Input: part model. Units: mm. Frame: model coordinates. A direction names the side the tool comes from. Give positions to 0.01 mm unless a question says otherwise; leave off trailing zeros. Loops run counter-clockwise (first coordinate to the right, second up) from the corner with the lowest first, then second, coordinate; pieces in that order, holes last. Notation, with made-up numbers: M -15.5,-6 L 34.5,-6 A24 ccw 34.5,4 Z; hole C 81,-32.75 d5. An arc over 180 degrees is marked long. Answer as a JSON object with one key per item and string values. Group by question number.
1) Section query B-B on y = 16.5. Return loops of the section in (x, z).
2) Section query C-C on z = -11. Return loops of the section in (x, y), plus the area to 3 significant figures.
3) Access query for faces 4 (the flat face through (11, 35, 0)), 5 (the flat face through (1, 35, -11)). Directions: +Z, -Z, +X, -X, +Y, -Y. A direction counts if a zero-diameter tool reaches every point of the face in a straight line with its end or side. Return the directions, or none.
4) Ray query, L1, parallel to Y at x = 11, z = -0.8; L2, parallel to X at y = 29.5, z = -7.75; L3, parallel to Z at x = 15.5, y = 45.5. Return the intervals inside material, ascending.
5) Section query D-D on z = -6. Return loops of the section in (x, y), plus the area to 3 significant figures.
6) Section query A-A on x = 11. Return loops of the section in (y, z).
7) Draft query along Z for faces 1 (the cylindrical face through (0.507, 18.483, -10.74)), 2 (the flat face through (11, 35, -1)), 3 (the flat face through (5.9, 70, -0.4)). Return one class per face: +Z half, -Z half, draft (parallel to the pull), parting line (faces both ways), or undercut.
8) First-contact query: P1, Ø5, axis at x = 11, y = 6.5, coming from the +Z side; P2, Ø6.5, axis at x = 11, y = 63.5, coming from the -Z side; P3, Ø1.5, axis at y = 11.5, z = -7, coming from the +X side. Flat tips, straight axial feed; report the tip coordinate or a pass-through.
from build123d import *

# Parameters (mm, degrees)
EXTRUSION1_DEPTH = 70
EXTRUSION2_REACH = 3
ESQUISSE2_R      = 2
EXTRUSION3_REACH = 3
ESQUISSE3_R      = 2


with BuildPart() as part:
    # Esquisse1 → Extrusion1 (new body)
    with BuildSketch(Plane(origin=(0, 0, 0), x_dir=(1, 0, 0), z_dir=(0, 1, 0))):
        Polygon((0, 0), (0, 21), (1, 21), (1, 1), (21, 1), (21, 0), align=None)
    extrude(amount=EXTRUSION1_DEPTH)

    # Esquisse2 → Extrusion2 (cut, up to next)
    with BuildSketch(Plane(origin=(1, 0, 0), x_dir=(0, 0, -1), z_dir=(1, 0, 0)), mode=Mode.PRIVATE) as extrusion2_sk1:
        with Locations((11, 16.5)):
            Circle(ESQUISSE2_R)
    extrusion2_tool1 = extrude(extrusion2_sk1.sketch, amount=-EXTRUSION2_REACH, mode=Mode.PRIVATE) & part.part
    add(extrusion2_tool1.solids().sort_by_distance((1, 16.5, -11))[0], mode=Mode.SUBTRACT)
    # Esquisse2 → Extrusion2 (cut, up to next)
    with BuildSketch(Plane(origin=(1, 0, 0), x_dir=(0, 0, -1), z_dir=(1, 0, 0)), mode=Mode.PRIVATE) as extrusion2_sk2:
        with Locations((11, 6.5)):
            Circle(ESQUISSE2_R)
    extrusion2_tool2 = extrude(extrusion2_sk2.sketch, amount=-EXTRUSION2_REACH, mode=Mode.PRIVATE) & part.part
    add(extrusion2_tool2.solids().sort_by_distance((1, 6.5, -11))[0], mode=Mode.SUBTRACT)
    # Esquisse2 → Extrusion2 (cut, up to next)
    with BuildSketch(Plane(origin=(1, 0, 0), x_dir=(0, 0, -1), z_dir=(1, 0, 0)), mode=Mode.PRIVATE) as extrusion2_sk3:
        with Locations((11, 53.5)):
            Circle(ESQUISSE2_R)
    extrusion2_tool3 = extrude(extrusion2_sk3.sketch, amount=-EXTRUSION2_REACH, mode=Mode.PRIVATE) & part.part
    add(extrusion2_tool3.solids().sort_by_distance((1, 53.5, -11))[0], mode=Mode.SUBTRACT)
    # Esquisse2 → Extrusion2 (cut, up to next)
    with BuildSketch(Plane(origin=(1, 0, 0), x_dir=(0, 0, -1), z_dir=(1, 0, 0)), mode=Mode.PRIVATE) as extrusion2_sk4:
        with Locations((11, 63.5)):
            Circle(ESQUISSE2_R)
    extrusion2_tool4 = extrude(extrusion2_sk4.sketch, amount=-EXTRUSION2_REACH, mode=Mode.PRIVATE) & part.part
    add(extrusion2_tool4.solids().sort_by_distance((1, 63.5, -11))[0], mode=Mode.SUBTRACT)

    # Esquisse3 → Extrusion3 (cut, up to next)
    with BuildSketch(Plane(origin=(0, 0, -1), x_dir=(-1, 0, 0), z_dir=(0, 0, -1)), mode=Mode.PRIVATE) as extrusion3_sk1:
        with Locations((-11, 53.5)):
            Circle(ESQUISSE3_R)
    extrusion3_tool1 = extrude(extrusion3_sk1.sketch, amount=-EXTRUSION3_REACH, mode=Mode.PRIVATE) & part.part
    add(extrusion3_tool1.solids().sort_by_distance((11, 53.5, -1))[0], mode=Mode.SUBTRACT)
    # Esquisse3 → Extrusion3 (cut, up to next)
    with BuildSketch(Plane(origin=(0, 0, -1), x_dir=(-1, 0, 0), z_dir=(0, 0, -1)), mode=Mode.PRIVATE) as extrusion3_sk2:
        with Locations((-11, 63.5)):
            Circle(ESQUISSE3_R)
    extrusion3_tool2 = extrude(extrusion3_sk2.sketch, amount=-EXTRUSION3_REACH, mode=Mode.PRIVATE) & part.part
    add(extrusion3_tool2.solids().sort_by_distance((11, 63.5, -1))[0], mode=Mode.SUBTRACT)
    # Esquisse3 → Extrusion3 (cut, up to next)
    with BuildSketch(Plane(origin=(0, 0, -1), x_dir=(-1, 0, 0), z_dir=(0, 0, -1)), mode=Mode.PRIVATE) as extrusion3_sk3:
        with Locations((-11, 6.5)):
            Circle(ESQUISSE3_R)
    extrusion3_tool3 = extrude(extrusion3_sk3.sketch, amount=-EXTRUSION3_REACH, mode=Mode.PRIVATE) & part.part
    add(extrusion3_tool3.solids().sort_by_distance((11, 6.5, -1))[0], mode=Mode.SUBTRACT)
    # Esquisse3 → Extrusion3 (cut, up to next)
    with BuildSketch(Plane(origin=(0, 0, -1), x_dir=(-1, 0, 0), z_dir=(0, 0, -1)), mode=Mode.PRIVATE) as extrusion3_sk4:
        with Locations((-11, 16.5)):
            Circle(ESQUISSE3_R)
    extrusion3_tool4 = extrude(extrusion3_sk4.sketch, amount=-EXTRUSION3_REACH, mode=Mode.PRIVATE) & part.part
    add(extrusion3_tool4.solids().sort_by_distance((11, 16.5, -1))[0], mode=Mode.SUBTRACT)


solid = part.part
Output:
{
 "1": {"outline": "M 0,-21 L 1,-21 L 1,-13 L 0,-13 Z; M 0,-9 L 1,-9 L 1,-1 L 9,-1 L 9,0 L 0,0 Z; M 13,-1 L 21,-1 L 21,0 L 13,0 Z"},
 "2": {"outline": "M 0,0 L 1,0 L 1,4.5 L 0,4.5 Z; M 0,8.5 L 1,8.5 L 1,14.5 L 0,14.5 Z; M 0,18.5 L 1,18.5 L 1,51.5 L 0,51.5 Z; M 0,55.5 L 1,55.5 L 1,61.5 L 0,61.5 Z; M 0,65.5 L 1,65.5 L 1,70 L 0,70 Z", "area": "54.0 mm^2"},
 "3": {"face 4": "+Z, +X, -X, +Y, -Y", "face 5": "-Z, +X, +Y, -Y"},
 "4": {"L1": "y = 0 to 4.5, 8.5 to 14.5, 18.5 to 51.5, 55.5 to 61.5, 65.5 to 70", "L2": "x = 0 to 1", "L3": "z = -1 to 0"},
 "5": {"outline": "M 0,0 L 1,0 L 1,70 L 0,70 Z", "area": "70.0 mm^2"},
 "6": {"outline": "M 0,-1 L 4.5,-1 L 4.5,0 L 0,0 Z; M 8.5,-1 L 14.5,-1 L 14.5,0 L 8.5,0 Z; M 18.5,-1 L 51.5,-1 L 51.5,0 L 18.5,0 Z; M 55.5,-1 L 61.5,-1 L 61.5,0 L 55.5,0 Z; M 65.5,-1 L 70,-1 L 70,0 L 65.5,0 Z"},
 "7": {"face 1": "undercut", "face 2": "-Z half", "face 3": "draft"},
 "8": {"P1": "stops at z = 0", "P2": "stops at z = -1", "P3": "stops at x = 1"}
}
